Check sheet for the modelled part. Datum: model origin and axes. Units: mm. A direction names the side the tool comes from. Coordinates: 2 decimals unless noted, no trailing zeros. Order: outer loops, then holes, each group sorted by start corner. A loop starts at its lowest first (then second) coordinate and runs counter-clockwise, first axis right, second up.
1. Draft check along X on faces 1 (the cylindrical face through (1.268, 53.692, -11.923)), 2 (the flat face through (110, -62, -17)), 3 (the flat face through (243, 81, 8)), 4 (the flat face through (10, -29, 9)). Enter one of: released by +X, released by -X, zero draft, split by the parting line, or undercut.
2. Cross-section at A-A (x = 70.5). Enter the section's corners in (y, z), then the cut area to 3 significant figures.
3. Cross-section at B-B (x = 41). Enter the section's corners in (y, z), then the cut area to 3 significant figures.
4. Gauge pin test, flat ends, axial feed: pin 1 Ø2 at (x, y) = (128.5, -82) entering from +Z; pin 2 Ø3.5 at (y, z) = (87.5, 28.43) entering from +X; pin 3 Ø10 at (y, z) = (19.5, 26) entering from +X; pin 4 Ø1 at (x, z) = (214, -55) entering from +Y. Record the tip position at first contact, or that the pin passes through.
5. Set-up check for faces 5 (the flat face through (57.5, -13, -25)), 6 (the cylindrical face through (4.93, 1.32, -29.97)), 7 (the flat face through (0, 24, 24)): record each of +Z, -Z, +X, -X, +Y, -Y from which the full face is reachable in a straight line by a thin tool's end or side.
6. Thickness scan on line 1 (Z direction, x = 7, y = 0); line 2 (X direction, y = 27, z = -18); line 3 (X direction, y = 16.5, z = -51.5). Record the ranges inside material, lowest first.
Autodesk Fusion 360 part; units mm, degrees
sketch "Sketch1" plane through (0, 0, 0) normal (0, 1, 0) x (1, 0, 0)
  line L0 (0, 0) -> (253, 0) construction
  line L1 (253, 0) -> (253, -120) construction
  line L2 (0, -120) -> (0, 0) construction
  line L3 (0, -55) -> (2.5, -55)
  line L4 (2.5, -55) -> (2.5, -53)
  line L5 (2.5, -53) -> (22.5, -53)
  line L6 (22.5, -53) -> (22.5, -55)
  line L7 (22.5, -55) -> (25, -55)
  line L8 (22.5, -55) -> (57.5, -55) construction
  line L9 (57.5, -55) -> (57.5, -30) construction
  line L10 (57.5, -30) -> (55, -30)
  line L11 (25, -55) -> (55, -30)
  line L12 (57.5, -30) -> (57.5, -29.7796)
  line L13 (57.5, -29.7796) -> (57.5, -28)
  line L14 (57.5, -28) -> (77.5, -28)
  line L15 (77.5, -28) -> (77.5, -30)
  line L16 (77.5, -30) -> (80, -30)
  line L17 (253, -120) -> (250, -120)
  line L18 (0, -55) -> (0, -30)
  arc A0 (87.5, -23.2906) -> (243, -109.7053) centre (255.0428, 95.0809) ccw
  line L19 (23.7795, -43) -> (51.1319, -20.2063)
  line L20 (10, -43) -> (23.7795, -43)
  line L21 (10, -43) -> (10, -30)
  line L22 (10, -30) -> (0, -30)
  line L23 (51.1319, -20.2063) -> (85.3629, -20.2063)
  line L24 (253, -120) -> (253, -110)
  arc A1 (85.3629, -20.2063) -> (243, -109.7053) centre (255.0428, 95.0809) ccw
  line L25 (253, -110) -> (253, -80)
  line L26 (253, -80) -> (243, -80)
  line L27 (243, -80) -> (243, -109.7053)
  line L28 (230, -118.5966) -> (230, -117.5)
  line L29 (230, -117.5) -> (250, -117.5)
  line L30 (250, -117.5) -> (250, -120)
  line L31 (253, -120) -> (250, -120) construction
  line L32 (230, -120) -> (0, -120) construction
  line L33 (190, -167.9989) -> (190, 64.1278) construction
  line L34 (170, -159.3868) -> (170, 52.862) construction
  line L35 (130, -158.4855) -> (130, 61.424) construction
  line L36 (110, -157.8306) -> (110, 88.7531) construction
  line L37 (358.5261, -104.57) -> (17.8717, -104.57) construction
  line L38 (363.4901, -75.89) -> (29.0407, -75.89) construction
  line L39 (170, -102.5373) -> (170, -104.57)
  line L40 (190, -104.57) -> (170, -104.57)
  arc A2 (190, -109.9914) -> (230, -118.5966) centre (255.0428, 95.0809) ccw
  line L41 (190, -109.9914) -> (190, -104.57)
  line L42 (110, -75.89) -> (130, -75.89)
  line L43 (110, -63.8147) -> (110, -75.89)
  line L44 (130, -75.89) -> (130, -79.9891)
  arc A3 (80, -30) -> (110, -63.8147) centre (255.0428, 95.0809) ccw
  arc A4 (130, -79.9891) -> (170, -102.5373) centre (255.0428, 95.0809) ccw
  dimension "d78" = 120
  dimension "d79" = 253
  dimension "d80" = 55
  dimension "d81" = 2.5
  dimension "d82" = 20
  dimension "d83" = 2
  dimension "d84" = 2
  dimension "d85" = 2.5
  dimension "d86" = 35
  dimension "d87" = 25
  dimension "d88" = 2.5
  dimension "d89" = 20
  dimension "d90" = 2
  dimension "d91" = 2
  dimension "d92" = 2.5
  dimension "d93" = 3
  dimension "d94" = 215.14
  dimension "d95" = 25
  dimension "d97" = 7.7937
  dimension "d98" = 80
  dimension "d99" = 10
  dimension "d100" = 20
  dimension "d101" = 2.5
  dimension "d102" = 40
  dimension "d103" = 20
  dimension "d104" = 40
  dimension "d105" = 20
  dimension "d106" = 75.89
  dimension "d107" = 104.57
revolve "Revolve3" add sketch "Sketch1" angle 360 about axis through (0, 0, 0) along (1, 0, 0)
sketch "Sketch6" plane through (253, 0, 0) normal (1, 0, 0) x (0, 1, 0)
  circle A0 centre (0, 0) radius 80
  circle A1 centre (0, 0) radius 120
  line L0 (0, 0) -> (0, 205.4416) construction
  circle A2 centre (0, 92) radius 2
  dimension "d109" = 4
  dimension "d110" = 92
extrude "Extrude3" cut sketch "Sketch6" along normal mid plane 30 contours A2
pattern_circular "C-Pattern3" count 10 over 360 about axis through (1.75, 0, 0) along (1, 0, 0) of "Extrude3"
sketch "Sketch7" plane through (0, 0, 0) normal (-1, 0, 0) x (0, -1, 0)
  circle A0 centre (0, 0) radius 55
  circle A1 centre (0, 0) radius 30
  line L0 (0, 0) -> (0, 179.9785) construction
  circle A2 centre (0, 47.5) radius 2
  dimension "d115" = 4
  dimension "d116" = 47.5
extrude "Extrude4" cut sketch "Sketch7" along normal mid plane 20 contours A2
pattern_circular "C-Pattern4" count 10 over 360 about axis through (1.75, 0, 0) along (1, 0, 0) of "Extrude4"
Data:
1. face 1: zero draft
1. face 2: released by -X
1. face 3: undercut
1. face 4: undercut
2. outline: circle Ø56 at (0, 0); hole circle Ø40.41 at (0, 0)
2. area: 1,180 mm2
3. outline: circle Ø83.33 at (0, 0); hole circle Ø57.3 at (0, 0)
3. area: 2,880 mm2
4. pin 1: passes through
4. pin 2: stops at x = 174.89
4. pin 3: stops at x = 98.5
4. pin 4: stops at y = 102.54
5. face 5: none
5. face 6: -X
5. face 7: +Z, -Z, -X, +Y, -Y
6. line 1: z = -53 to -49.5, -45.5 to -30, 30 to 45.5, 49.5 to 53
6. line 2: x = 0 to 10, 36.44 to 52.06, 81.78 to 94.36
6. line 3: x = 0 to 2.5, 22.5 to 26.11, 100.01 to 114.21
